Source: CAD feature listing. Evaluate the final solid. Frame: model axes, mm. A direction names the side the tool comes from. Give positions to 0.01 mm unless a question says otherwise; leave off trailing zeros. Loops run counter-clockwise (first coordinate to the right, second up) from the corner with the lowest first, then second, coordinate; pieces in that order, holes last. Notation, with made-up numbers: (-8.5, 49.25) - (37.5, 49.25) arc R26 cw to (37.5, 82.25) - close; hole circle Ø10 at (52.25, -29). An arc over 180 degrees is marked (long way). Write each question's results on one line, items separated by ' | '. Start each with the question number.
(1) Material intervals for line 1 along X through (y, z) = (318, 58.5); line 2 along Z through (x, y) = (-239, 260); line 3 along Y through (x, z) = (-114, 25), sorted ascending. Write a range as [from, to].
(2) Cut plane D-D on z = 25. Return the cut outline in (x, y).
(3) Reachability of faces 5 (the flat face through (-109.697, 241, 74)), 6 (the flat face through (-99.697, 240, 74)), 7 (the flat face through (-278.14, 96.485, 73.95)) from +Z, -Z, +X, -X, +Y, -Y: full face, straight path, thin tool, end or side. Return the list, or none.
(4) Pull-direction query (Z, two-part tool) for faces 1 (the cylindrical face through (-336.805, 5.127, 76.05)), 2 (the flat face through (-161, 6, 0)), 3 (the cylindrical face through (-104.8, 230.1, 34.5)), 4 (the cylindrical face through (-240.767, 236.544, 127.498)); classes: pulls with the +Z half, pulls with the -Z half, needs draft (parallel to the pull), parting line crosses it, or undercut.
(5) Cut plane A-A on y = 260. Return the cut outline in (x, z), then the cut area to 3 significant figures.
(6) Contact query for flat-ended pins moving along their axis: pin 1 (2 mm diameter, centred on x = -78, z = 18.5, fed in from +Y); pin 2 (5 mm diameter, centred on y = 43.5, z = 83, fed in from +X); pin 3 (4 mm diameter, centred on x = -205.5, z = 66, fed in from -Y); pin 4 (6 mm diameter, centred on y = 176.5, z = 50.5, fed in from -X). Output: stop coordinate, or through.
(7) Cut plane B-B on x = -88.5. Return the cut outline in (y, z).
(8) Cut plane C-C on y = 310. Return the cut outline in (x, z).
from build123d import *

# Parameters (mm, degrees)
SALIENTE_EXTRUIR1_DEPTH = 150
CROQUIS2_R              = 7.5
CORTAR_EXTRUIR1_DEPTH   = 146
REDONDEO1_R             = 75
REDONDEO2_R             = 10


with BuildPart() as part:
    # Croquis1 → Saliente-Extruir1 (new body)
    with BuildSketch(Plane.XY):
        Polygon((-245.696551146, 350), (-245.696551146, 172.679491924), (-345.393102292, 0), (0, 0), (-99.696551146, 172.679491924), (-99.696551146, 350), (-109.696551146, 350), (-109.696551146, 170), (-17.320508076, 10), (-328.072594216, 10), (-235.696551146, 170), (-235.696551146, 350), align=None)
    extrude(amount=SALIENTE_EXTRUIR1_DEPTH)

    # Croquis2 → Cortar-Extruir1 (cut)
    with BuildSketch(Plane.ZY.offset(245.696551146)):
        with Locations(Location((75, 260, 0), (0, 0, 270))):
            Circle(CROQUIS2_R)
        with BuildLine():
            ThreePointArc((34.341360082, 219.341360082), (128.123073119, 237.995702639), (75, 317.5))
            ThreePointArc((75, 317.5), (67.5, 310), (75, 302.5))
            ThreePointArc((75, 302.5), (114.264880132, 243.735954124), (44.9479618, 229.9479618))
            ThreePointArc((44.9479618, 229.9479618), (34.341360082, 229.9479618), (34.341360082, 219.341360082))
        make_face()
    extrude(amount=-CORTAR_EXTRUIR1_DEPTH, mode=Mode.SUBTRACT)

    # Redondeo1
    redondeo1_edges = [part.edges().sort_by_distance(p)[0] for p in [
        (-104.696551146, 350, 0),
        (-104.696551146, 350, 150),
        (-240.696551146, 350, 150),
        (-240.696551146, 350, 0),
    ]]
    fillet(redondeo1_edges, radius=REDONDEO1_R - 0.0001)  # a hair under: the kernel refuses the full size

    # Redondeo2
    redondeo2_edges = [part.edges().sort_by_distance(p)[0] for p in [
        (-328.072594216, 10, 75),
        (-17.320508076, 10, 75),
        (0, 0, 75),
        (-345.393102292, 0, 75),
    ]]
    fillet(redondeo2_edges, radius=REDONDEO2_R)


solid = part.part
Ans:
1) line 1: [-245.7, -235.7], [-109.7, -99.7] | line 2: [0, 67.5], [82.5, 117.5], [132.5, 150] | line 3: [0, 10]
2) outline: (-336.73, 15) arc R10 ccw to (-328.07, 0) - (-17.32, 0) arc R10 ccw to (-8.66, 15) - (-99.7, 172.68) - (-99.7, 330.9) - (-109.7, 330.9) - (-109.7, 170) - (-25.98, 25) arc R10 cw to (-34.64, 10) - (-310.75, 10) arc R10 cw to (-319.41, 25) - (-235.7, 170) - (-235.7, 330.9) - (-245.7, 330.9) - (-245.7, 172.68) - close
3) face 5: +Z, -Z, +Y | face 6: +Z, -Z, +X, +Y | face 7: +Z, -Z
4) face 1: needs draft | face 2: pulls with the -Z half | face 3: undercut | face 4: undercut
5) outline: (-245.7, 0) - (-235.7, 0) - (-235.7, 67.5) - (-245.7, 67.5) - close; (-245.7, 82.5) - (-235.7, 82.5) - (-235.7, 117.5) - (-245.7, 117.5) - close; (-245.7, 132.5) - (-235.7, 132.5) - (-235.7, 150) - (-245.7, 150) - close; (-109.7, 0) - (-99.7, 0) - (-99.7, 67.5) - (-109.7, 67.5) - close; (-109.7, 82.5) - (-99.7, 82.5) - (-99.7, 117.5) - (-109.7, 117.5) - close; (-109.7, 132.5) - (-99.7, 132.5) - (-99.7, 150) - (-109.7, 150) - close | area: 2,400 mm^2
6) pin 1: y = 136.83 | pin 2: x = -23.67 | pin 3: y = 0 | pin 4: x = -245.7
7) outline: (0, 0) - (10, 0) - (10, 150) - (0, 150) - close; (133.29, 0) - (153.29, 0) - (153.29, 150) - (133.29, 150) - close
8) outline: (-245.7, 8.67) - (-235.7, 8.67) - (-235.7, 67.5) - (-245.7, 67.5) - close; (-245.7, 103.39) - (-235.7, 103.39) - (-235.7, 141.33) - (-245.7, 141.33) - close; (-109.7, 8.67) - (-99.7, 8.67) - (-99.7, 67.5) - (-109.7, 67.5) - close; (-109.7, 103.39) - (-99.7, 103.39) - (-99.7, 141.33) - (-109.7, 141.33) - close
